Read the model definition and answer for the solid it produces. Units are mm, in the model's axes. Coordinates: 2 decimals unless noted, no trailing zeros. Return JSON: item names as keys, results as strings.
```python
from build123d import *

# Parameters (mm, degrees)
F1_DEPTH = 240


# Not quite as in the source:
# - ends of sketch curves that miss each other by under 0.0002 mm in the source are joined


with BuildPart() as f1:
    # F0 (on Front) → F1 (new body)
    with BuildSketch(Plane.XZ):
        with BuildLine():
            ThreePointArc((0, 2.15), (1.5202795796, 1.5202795796), (2.15, 0))
            Line((2.15, 0), (3, 0))
            Line((3, 0), (3.307278, 0.307278))
            ThreePointArc((3.307278, 0.307278), (3.7143803747, 2.2820219924), (4.7078187099, 4.0365664363))
            ThreePointArc((4.7078187099, 4.0365664363), (4.812308461, 4.1201573706), (4.94275, 4.15))
            Line((4.94275, 4.15), (8.2, 4.15))
            ThreePointArc((8.2, 4.15), (8.4121320344, 4.0621320344), (8.5, 3.85))
            Line((8.5, 3.85), (8.5, 2.95))
            ThreePointArc((8.5, 2.95), (8.5878679656, 2.7378679656), (8.8, 2.65))
            Line((8.8, 2.65), (9.7, 2.65))
            ThreePointArc((9.7, 2.65), (9.9121320344, 2.7378679656), (10, 2.95))
            Line((10, 2.95), (10, 9.7))
            ThreePointArc((10, 9.7), (9.9121320344, 9.9121320344), (9.7, 10))
            Line((9.7, 10), (2.95, 10))
            ThreePointArc((2.95, 10), (2.7378679656, 9.9121320344), (2.65, 9.7))
            Line((2.65, 9.7), (2.65, 8.8))
            ThreePointArc((2.65, 8.8), (2.7378679656, 8.5878679656), (2.95, 8.5))
            Line((2.95, 8.5), (3.85, 8.5))
            ThreePointArc((3.85, 8.5), (4.0621320344, 8.4121320344), (4.15, 8.2))
            Line((4.15, 8.2), (4.15, 4.94275))
            ThreePointArc((4.15, 4.94275), (4.1201572004, 4.8123081084), (4.036566086, 4.7078178916))
            ThreePointArc((4.036566086, 4.7078178916), (2.2820216259, 3.7143802371), (0.3072779813, 3.3072783955))
            Line((0.3072779813, 3.3072783955), (0, 3))
            Line((0, 3), (0, 2.15))
        make_face()
        with BuildLine():
            ThreePointArc((7, 9), (8.4142135624, 8.4142135624), (9, 7))
            ThreePointArc((9, 7), (8.4142135624, 5.5857864376), (7, 5))
            ThreePointArc((7, 5), (5.5857864376, 5.5857864376), (5, 7))
            ThreePointArc((5, 7), (5.5857864376, 8.4142135624), (7, 9))
        make_face(mode=Mode.SUBTRACT)
        with BuildLine():
            Line((3, 0), (2.15, 0))
            ThreePointArc((2.15, 0), (1.5202795796, -1.5202795796), (0, -2.15))
            Line((0, -2.15), (0, -3))
            Line((0, -3), (0.307278, -3.307277))
            ThreePointArc((0.307278, -3.307277), (2.2820216259, -3.7143792371), (4.036565823, -4.7078172229))
            ThreePointArc((4.036565823, -4.7078172229), (4.1201572004, -4.8123071084), (4.15, -4.942749))
            Line((4.15, -4.942749), (4.15, -8.2))
            ThreePointArc((4.15, -8.2), (4.0621320344, -8.4121320344), (3.85, -8.5))
            Line((3.85, -8.5), (2.95, -8.5))
            ThreePointArc((2.95, -8.5), (2.7378679656, -8.5878679656), (2.65, -8.8))
            Line((2.65, -8.8), (2.65, -9.7))
            ThreePointArc((2.65, -9.7), (2.7378679656, -9.9121320344), (2.95, -10))
            Line((2.95, -10), (9.7, -10))
            ThreePointArc((9.7, -10), (9.9121320344, -9.9121320344), (10, -9.7))
            Line((10, -9.7), (10, -2.95))
            ThreePointArc((10, -2.95), (9.9121320344, -2.7378679656), (9.7, -2.65))
            Line((9.7, -2.65), (8.8, -2.65))
            ThreePointArc((8.8, -2.65), (8.5878679656, -2.7378679656), (8.5, -2.95))
            Line((8.5, -2.95), (8.5, -3.85))
            ThreePointArc((8.5, -3.85), (8.4121320344, -4.0621320344), (8.2, -4.15))
            Line((8.2, -4.15), (4.94275, -4.15))
            ThreePointArc((4.94275, -4.15), (4.8123081084, -4.1201572004), (4.7078178916, -4.036566086))
            ThreePointArc((4.7078178916, -4.036566086), (3.7143800615, -2.2820211583), (3.3072783483, -0.3072769835))
            Line((3.3072783483, -0.3072769835), (3, 0))
        make_face()
        with BuildLine():
            ThreePointArc((7, -5), (8.4142135624, -5.5857864376), (9, -7))
            ThreePointArc((9, -7), (8.4142135624, -8.4142135624), (7, -9))
            ThreePointArc((7, -9), (5.5857864376, -8.4142135624), (5, -7))
            ThreePointArc((5, -7), (5.5857864376, -5.5857864376), (7, -5))
        make_face(mode=Mode.SUBTRACT)
        with BuildLine():
            ThreePointArc((-2.15, 0), (-1.5202795796, 1.5202795796), (0, 2.15))
            Line((0, 2.15), (0, 3))
            Line((0, 3), (-0.307277, 3.307278))
            ThreePointArc((-0.307277, 3.307278), (-2.2820211583, 3.7143800615), (-4.036565823, 4.7078182229))
            ThreePointArc((-4.036565823, 4.7078182229), (-4.1201572004, 4.8123081084), (-4.15, 4.94275))
            Line((-4.15, 4.94275), (-4.15, 8.2))
            ThreePointArc((-4.15, 8.2), (-4.0621320344, 8.4121320344), (-3.85, 8.5))
            Line((-3.85, 8.5), (-2.95, 8.5))
            ThreePointArc((-2.95, 8.5), (-2.7378679656, 8.5878679656), (-2.65, 8.8))
            Line((-2.65, 8.8), (-2.65, 9.7))
            ThreePointArc((-2.65, 9.7), (-2.7378679656, 9.9121320344), (-2.95, 10))
            Line((-2.95, 10), (-9.7, 10))
            ThreePointArc((-9.7, 10), (-9.9121320344, 9.9121320344), (-10, 9.7))
            Line((-10, 9.7), (-10, 2.95))
            ThreePointArc((-10, 2.95), (-9.9121320344, 2.7378679656), (-9.7, 2.65))
            Line((-9.7, 2.65), (-8.8, 2.65))
            ThreePointArc((-8.8, 2.65), (-8.5878679656, 2.7378679656), (-8.5, 2.95))
            Line((-8.5, 2.95), (-8.5, 3.85))
            ThreePointArc((-8.5, 3.85), (-8.4121320344, 4.0621320344), (-8.2, 4.15))
            Line((-8.2, 4.15), (-4.942749, 4.15))
            ThreePointArc((-4.942749, 4.15), (-4.812307461, 4.1201573706), (-4.7078173786, 4.0365666993))
            ThreePointArc((-4.7078173786, 4.0365666993), (-3.7143793747, 2.2820219924), (-3.3072773955, 0.3072779813))
            Line((-3.3072773955, 0.3072779813), (-3, 0))
            Line((-3, 0), (-2.15, 0))
        make_face()
        with BuildLine():
            ThreePointArc((-7, 5), (-8.4142135624, 5.5857864376), (-9, 7))
            ThreePointArc((-9, 7), (-8.4142135624, 8.4142135624), (-7, 9))
            ThreePointArc((-7, 9), (-5.5857864376, 8.4142135624), (-5, 7))
            ThreePointArc((-5, 7), (-5.5857864376, 5.5857864376), (-7, 5))
        make_face(mode=Mode.SUBTRACT)
        with BuildLine():
            Line((0, -3), (0, -2.15))
            ThreePointArc((0, -2.15), (-1.5202795796, -1.5202795796), (-2.15, 0))
            Line((-2.15, 0), (-3, 0))
            Line((-3, 0), (-3.307277, -0.307277))
            ThreePointArc((-3.307277, -0.307277), (-3.7143790615, -2.2820211583), (-4.7078172229, -4.036565823))
            ThreePointArc((-4.7078172229, -4.036565823), (-4.8123071084, -4.1201572004), (-4.942749, -4.15))
            Line((-4.942749, -4.15), (-8.2, -4.15))
            ThreePointArc((-8.2, -4.15), (-8.4121320344, -4.0621320344), (-8.5, -3.85))
            Line((-8.5, -3.85), (-8.5, -2.95))
            ThreePointArc((-8.5, -2.95), (-8.5878679656, -2.7378679656), (-8.8, -2.65))
            Line((-8.8, -2.65), (-9.7, -2.65))
            ThreePointArc((-9.7, -2.65), (-9.9121320344, -2.7378679656), (-10, -2.95))
            Line((-10, -2.95), (-10, -9.7))
            ThreePointArc((-10, -9.7), (-9.9121320344, -9.9121320344), (-9.7, -10))
            Line((-9.7, -10), (-2.95, -10))
            ThreePointArc((-2.95, -10), (-2.7378679656, -9.9121320344), (-2.65, -9.7))
            Line((-2.65, -9.7), (-2.65, -8.8))
            ThreePointArc((-2.65, -8.8), (-2.7378679656, -8.5878679656), (-2.95, -8.5))
            Line((-2.95, -8.5), (-3.85, -8.5))
            ThreePointArc((-3.85, -8.5), (-4.0621320344, -8.4121320344), (-4.15, -8.2))
            Line((-4.15, -8.2), (-4.15, -4.942749))
            ThreePointArc((-4.15, -4.942749), (-4.1201572004, -4.8123071084), (-4.036566086, -4.7078168916))
            ThreePointArc((-4.036566086, -4.7078168916), (-2.2820211583, -3.7143790615), (-0.3072769835, -3.3072773483))
            Line((-0.3072769835, -3.3072773483), (0, -3))
        make_face()
        with BuildLine():
            ThreePointArc((-7, -9), (-8.4142135624, -8.4142135624), (-9, -7))
            ThreePointArc((-9, -7), (-8.4142135624, -5.5857864376), (-7, -5))
            ThreePointArc((-7, -5), (-5.5857864376, -5.5857864376), (-5, -7))
            ThreePointArc((-5, -7), (-5.5857864376, -8.4142135624), (-7, -9))
        make_face(mode=Mode.SUBTRACT)
    extrude(amount=F1_DEPTH)


solid = f1.part
```
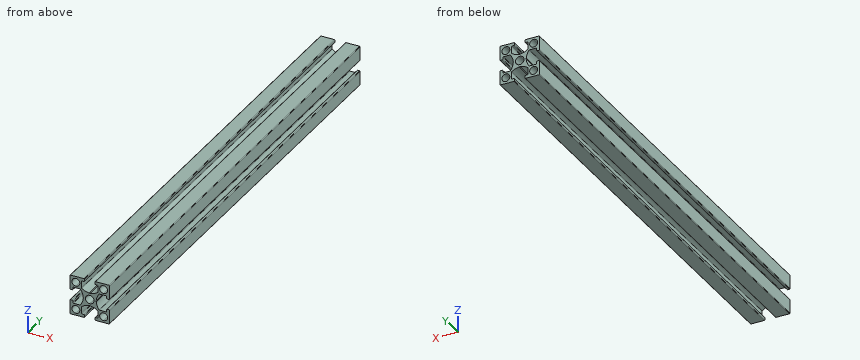
(1) Flat-ended cylindrical pins translate along their axes: P1, Ø10, axis at x = -8, z = -7, coming from the -Y side; P2, Ø1, axis at x = 7.5, z = -6, coming from the -Y side. Find the tip coordinate at first contact, or state that the pin passes through.
Answer:
{"P1": "y = -240", "P2": "through"}
(2) A cutting plane is placed at A-A (y = -143). State how many separate pieces and enclosed holes the cut face has, and give its area (3 significant figures).
Answer:
{"separate pieces": "1", "enclosed holes": "5", "area": "146 mm²"}
(3) Straight lines are drawn through the part: line 1 (X direction, y = -66.5, z = 6.75); line 2 (X direction, y = -140.5, z = 8.75). For each, find the intervals that lie inside material, in ascending order. Write a range as from..to.
Answer:
{"line 1": "-10..-8.98, -5.02..-4.15, 4.15..5.02, 8.98..10", "line 2": "-10..-7.97, -6.03..-2.65, 2.65..6.03, 7.97..10"}
